Can you work these out from the model? Positions are in its coordinate system, mm. Face numbers are marked on the shaded views. A direction names the side the tool comes from. Round coordinates to 2 decimals unless told otherwise and drop trailing zeros. Loops run counter-clockwise (first coordinate to the right, second up) from the corner with the lowest first, then second, coordinate; pieces in that order, holes last.
(1) I want a section at C-C on z = 0. Write out the boundary of the cut face in (x, y).
(2) I want a section at D-D on y = 36. Write out the boundary of the cut face in (x, z), plus the area to 3 significant figures.
(3) Thinking about a two-plate mould opening in Z: for the marked faces 4, 5, 6 and 7, which applies, released by +Z, released by -Z, zero draft, split by the parting line, or undercut?
(4) Will these pins go through, and if not, where does the flat tip stop? pin 1 Ø4 at (x, y) = (0.5, 45.5) entering from -Z; pin 2 Ø16 at (x, z) = (18.5, 14) entering from -Y; pin 3 Ø12.5 at (x, z) = (0.5, -1) entering from -Y; pin 4 Ø5 at (x, z) = (-18.5, -14) entering from -Y.
(5) Which directions (+Z, -Z, +X, -X, +Y, -Y) give clear straight access to the entire face, cutting with the end or side of a thin tool? Please do the marked faces 1, 2 and 3.
(6) If I drill on line 1 along Z through (x, y) = (0, 11.5); line 2 along Z through (x, y) = (-18.5, 46); line 3 along Z through (x, y) = (-18.5, 47.5), over which ranges is the centre line in solid material (lowest first)?
(7) I want a section at B-B on x = -18.5. Write out the boundary of the cut face in (y, z).
(8) I want a section at A-A on y = 44. Write out the boundary of the cut face in (x, z).
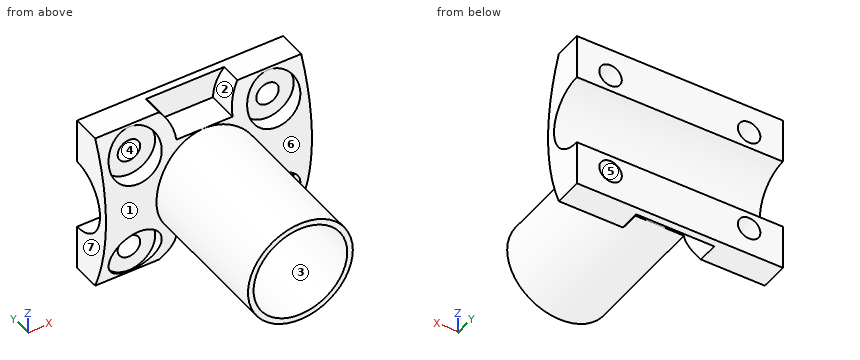
Solid Edge part; units mm, degrees
sketch "Sketch1" plane through (0, 50, 11.75) normal (0, -1, 0) x (1, 0, 0)
  line L0 (-27.5, -33.25) -> (27.5, -33.25)
  line L1 (27.5, 9.75) -> (27.5, -33.25)
  line L2 (27.5, 9.75) -> (-27.5, 9.75)
  line L3 (-27.5, 9.75) -> (-27.5, -33.25)
  dimension "D1" = 27.5
  dimension "D2" = 27.5
extrude "ExtrudedProtrusion_2" add sketch "Sketch1" along normal blind 12
sketch "Sketch2" plane through (0, 0, 0) normal (1, 0, 0) x (0, 1, 0)
  arc A0 (50, -9.5) -> (50, 9.5) centre (50, 0) cw
  line L0 (50, 9.5) -> (50, -9.5)
  dimension "D1" = 50
extrude "Cutout1" cut sketch "Sketch2" along normal through all and the other way through all
sketch "Sketch3" plane through (-27.5, 44, 0) normal (-1, 0, 0) x (0, 0, -1)
  line L0 (-21.5, -6) -> (-21.5, 1.5)
  arc A0 (-21.5, 1.5) -> (21.5, 1.5) centre (0, -48.0353) cw
  line L1 (21.5, -6) -> (21.5, 1.5)
  line L2 (27.9876, -6) -> (21.5, -6)
  line L3 (27.9876, 18.1819) -> (27.9876, -6)
  line L4 (-27.4197, 18.1819) -> (27.9876, 18.1819)
  line L5 (-27.4197, -6) -> (-27.4197, 18.1819)
  line L6 (-21.5, -6) -> (-27.4197, -6)
extrude "Cutout2" cut sketch "Sketch3" against normal up to next
sketch "Sketch4" plane through (0, 0, 0) normal (0, -1, 0) x (1, 0, 0)
  circle A0 centre (0, 0) radius 14
extrude "Protrusion1" add sketch "Sketch4" against normal up to next
sketch "Sketch5" plane through (0, 0, 0) normal (0, -1, 0) x (1, 0, 0)
  circle A0 centre (0, 0) radius 12.5
extrude "Cutout3" cut sketch "Sketch5" against normal blind 37
sketch "Sketch6" plane through (0, 38, 0) normal (0, -1, 0) x (1, 0, 0)
  circle A0 centre (-18.5, -14) radius 3
  circle A1 centre (18.5, -14) radius 3
  circle A2 centre (18.5, 14) radius 3
  circle A3 centre (-18.5, 14) radius 3
  dimension "D1" = 18.5
  dimension "D2" = 18.5
extrude "Cutout4" cut sketch "Sketch6" against normal through all
sketch "Sketch7" plane through (0, 38, 0) normal (0, -1, 0) x (1, 0, 0)
  circle A0 centre (-18.5, 14) radius 7
  circle A1 centre (18.5, 14) radius 7
  circle A2 centre (-18.5, -14) radius 7
  circle A3 centre (18.5, -14) radius 7
extrude "ExtrudedCutout_8" cut sketch "Sketch7" against normal blind 4.5
sketch "Sketch8" plane through (0, 38, 0) normal (0, -1, 0) x (1, 0, 0)
  arc A0 (10.4533, -21.5) -> (7.5, -14) centre (18.5, -14) cw
  line L0 (-7.5, -14) -> (7.5, -14)
  arc A1 (-10.4533, -21.5) -> (-7.5, -14) centre (-18.5, -14) ccw
  line L1 (-10.4533, -21.5) -> (10.4533, -21.5)
  line L2 (-10.4533, 21.5) -> (10.4533, 21.5)
  arc A2 (7.5, 14) -> (10.4533, 21.5) centre (18.5, 14) cw
  line L3 (-7.5, 14) -> (7.5, 14)
  arc A3 (-7.5, 14) -> (-10.4533, 21.5) centre (-18.5, 14) ccw
  dimension "D1" = 7.5
extrude "ExtrudedCutout_9" cut sketch "Sketch8" against normal blind 10
properties material "Aluminum, 1060"
Filled sheet:
1. outline: (-27.5, 38.04) - (-14, 38.04) - (-14, 0) - (-12.5, 0) - (-12.5, 37) - (12.5, 37) - (12.5, 0) - (14, 0) - (14, 38.04) - (27.5, 38.04) - (27.5, 40.5) - (-27.5, 40.5) - close
2. outline: circle Ø28 at (0, 0); hole circle Ø25 at (0, 0)
2. area: 125 mm2
3. face 4: undercut
3. face 5: undercut
3. face 6: split by the parting line
3. face 7: zero draft
4. pin 1: stops at z = -14
4. pin 2: stops at y = 38.37
4. pin 3: stops at y = 37
4. pin 4: passes through
5. face 1: -X, -Y
5. face 2: +Z, -Y
5. face 3: -Y
6. line 1: z = -14 to -12.5, 12.5 to 14
6. line 2: z = -21.5 to -17, -11 to -8.62, 8.62 to 11, 17 to 21.5
6. line 3: z = -21.5 to -17, -11 to -9.17, 9.17 to 11, 17 to 21.5
7. outline: (38.49, -7) - (42.5, -7) - (42.5, -11) - (50, -11) - (50, -9.5) arc R9.5 cw to (50, 9.5) - (50, 11) - (42.5, 11) - (42.5, 7) - (38.49, 7) arc R54 ccw to start; (42.29, -21) arc R54 ccw to (42.5, -21.5) - (50, -21.5) - (50, -17) - (42.5, -17) - (42.5, -21) - close; (42.29, 21) - (42.5, 21) - (42.5, 17) - (50, 17) - (50, 21.5) - (42.5, 21.5) arc R54 ccw to start
8. outline: (-27.5, -21.5) - (-10.45, -21.5) arc R11 ccw to (-7.5, -14) - (7.5, -14) arc R11 ccw to (10.45, -21.5) - (27.5, -21.5) - (27.5, -7.37) - (-27.5, -7.37) - close; (-27.5, 7.37) - (27.5, 7.37) - (27.5, 21.5) - (10.45, 21.5) arc R11 ccw to (7.5, 14) - (-7.5, 14) arc R11 ccw to (-10.45, 21.5) - (-27.5, 21.5) - close; hole circle Ø6 at (-18.5, -14); hole circle Ø6 at (-18.5, 14); hole circle Ø6 at (18.5, -14); hole circle Ø6 at (18.5, 14)
